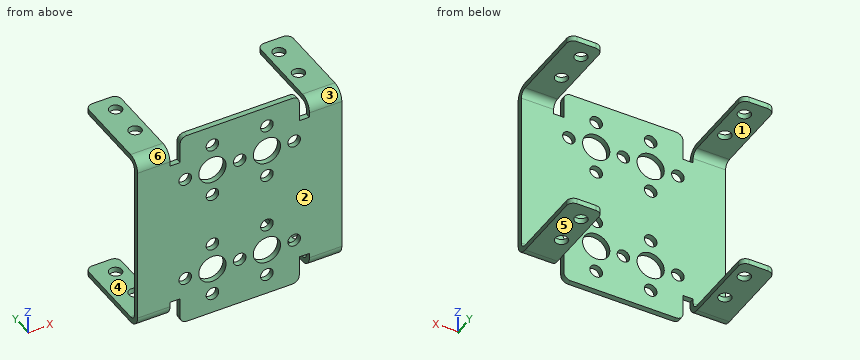
from build123d import *

# Parameters (mm, degrees)
BASE_FLANGE1_DEPTH             = 1.6
EDGE_FLANGE1_STRIP_W           = 10.4
EDGE_FLANGE1_STRIP_H           = 1.6
EDGE_FLANGE1_STRIP_CUT_DEPTH   = 9.5
EDGE_FLANGE1_STRIP_2_W         = 10.4
EDGE_FLANGE1_STRIP_2_H         = 1.6
EDGE_FLANGE1_STRIP_CUT_2_DEPTH = 9.5
EDGE_FLANGE1_DEPTH             = 9.5
EDGE_FLANGE1_BEND_DEPTH        = 9.5
CUT_EXTRUDE1_REACH             = 51.346
SKETCH15_R                     = 1.85
SKETCH15_R_2                   = 4
CUT_EXTRUDE2_REACH             = 50.448
SKETCH16_R                     = 1.85
FILLET1_R                      = 2


# Sheet-metal steps are written as plain solids
with BuildPart() as part:
    # Sketch1 → Base-Flange1 (new body)
    with BuildSketch(Plane(origin=(0, 0, 0), x_dir=(1, 0, 0), z_dir=(0, 1, 0))):
        Polygon((-30, 0), (30, 0), (30, -27), (20.5, -27), (20.5, -22), (17.5, -22), (17.5, -30), (-17.5, -30), (-17.5, -22), (-20.5, -22), (-20.5, -27), (-30, -27), align=None)
    extrude(amount=BASE_FLANGE1_DEPTH)

    # Edge-Flange1 strip (across the edge) → Edge-Flange1 strip cut (cut)
    with BuildSketch(Plane(origin=(20.5, 1.6, 27), x_dir=(0, 0, -1), z_dir=(1, 0, 0))):
        with Locations((-1.6, -0.8)):
            Rectangle(EDGE_FLANGE1_STRIP_W, EDGE_FLANGE1_STRIP_H)
    extrude(amount=EDGE_FLANGE1_STRIP_CUT_DEPTH, mode=Mode.SUBTRACT)

    # Edge-Flange1 strip 2 (across the edge) → Edge-Flange1 strip cut 2 (cut)
    with BuildSketch(Plane(origin=(-30, 1.6, 27), x_dir=(0, 0, -1), z_dir=(1, 0, 0))):
        with Locations((-1.6, -0.8)):
            Rectangle(EDGE_FLANGE1_STRIP_2_W, EDGE_FLANGE1_STRIP_2_H)
    extrude(amount=EDGE_FLANGE1_STRIP_CUT_2_DEPTH, mode=Mode.SUBTRACT)

    # Edge-Flange1 section (across the edge) → Edge-Flange1 (add)
    with BuildSketch(Plane(origin=(20.5, 1.6, 27), x_dir=(0, 0, -1), z_dir=(1, 0, 0))):
        with BuildLine():
            Line((0, 2), (0, 25.2))
            Line((0, 25.2), (1.6, 25.2))
            Line((1.6, 25.2), (1.6, 2))
            ThreePointArc((1.6, 2), (2.185786438, 0.585786438), (3.6, 0))
            Line((3.6, 0), (3.6, -1.6))
            ThreePointArc((3.6, -1.6), (1.054415588, -0.545584412), (0, 2))
        make_face()
    extrude(amount=EDGE_FLANGE1_DEPTH)

    # Edge-Flange1 section 2 (across the edge) → Edge-Flange1 bend (add)
    with BuildSketch(Plane(origin=(-30, 1.6, 27), x_dir=(0, 0, -1), z_dir=(1, 0, 0))):
        with BuildLine():
            Line((0, 2), (0, 25.2))
            Line((0, 25.2), (1.6, 25.2))
            Line((1.6, 25.2), (1.6, 2))
            ThreePointArc((1.6, 2), (2.185786438, 0.585786438), (3.6, 0))
            Line((3.6, 0), (3.6, -1.6))
            ThreePointArc((3.6, -1.6), (1.054415588, -0.545584412), (0, 2))
        make_face()
    extrude(amount=EDGE_FLANGE1_BEND_DEPTH)

    # Sketch15 → Cut-Extrude1 (cut, up to next)
    with BuildSketch(Plane(origin=(0, 1.6, 0), x_dir=(1, 0, 0), z_dir=(0, 1, 0)), mode=Mode.PRIVATE) as cut_extrude1_sk1:
        with Locations(Location((0, -16, 0), (0, 0, 270))):
            Circle(SKETCH15_R)
    cut_extrude1_tool1 = extrude(cut_extrude1_sk1.sketch, amount=-CUT_EXTRUDE1_REACH, mode=Mode.PRIVATE) & part.part
    # Sketch15 → Cut-Extrude1 (cut, up to next)
    with BuildSketch(Plane(origin=(0, 1.6, 0), x_dir=(1, 0, 0), z_dir=(0, 1, 0)), mode=Mode.PRIVATE) as cut_extrude1_sk2:
        with Locations(Location((8, -16, 0), (0, 0, 270))):
            Circle(SKETCH15_R_2)
    cut_extrude1_tool2 = extrude(cut_extrude1_sk2.sketch, amount=-CUT_EXTRUDE1_REACH, mode=Mode.PRIVATE) & part.part
    # Sketch15 → Cut-Extrude1 (cut, up to next)
    with BuildSketch(Plane(origin=(0, 1.6, 0), x_dir=(1, 0, 0), z_dir=(0, 1, 0)), mode=Mode.PRIVATE) as cut_extrude1_sk3:
        with Locations(Location((-8, -16, 0), (0, 0, 270))):
            Circle(SKETCH15_R_2)
    cut_extrude1_tool3 = extrude(cut_extrude1_sk3.sketch, amount=-CUT_EXTRUDE1_REACH, mode=Mode.PRIVATE) & part.part
    # Sketch15 → Cut-Extrude1 (cut, up to next)
    with BuildSketch(Plane(origin=(0, 1.6, 0), x_dir=(1, 0, 0), z_dir=(0, 1, 0)), mode=Mode.PRIVATE) as cut_extrude1_sk4:
        with Locations(Location((16, -16, 0), (0, 0, 270))):
            Circle(SKETCH15_R)
    cut_extrude1_tool4 = extrude(cut_extrude1_sk4.sketch, amount=-CUT_EXTRUDE1_REACH, mode=Mode.PRIVATE) & part.part
    # Sketch15 → Cut-Extrude1 (cut, up to next)
    with BuildSketch(Plane(origin=(0, 1.6, 0), x_dir=(1, 0, 0), z_dir=(0, 1, 0)), mode=Mode.PRIVATE) as cut_extrude1_sk5:
        with Locations(Location((-16, -16, 0), (0, 0, 270))):
            Circle(SKETCH15_R)
    cut_extrude1_tool5 = extrude(cut_extrude1_sk5.sketch, amount=-CUT_EXTRUDE1_REACH, mode=Mode.PRIVATE) & part.part
    # Sketch15 → Cut-Extrude1 (cut, up to next)
    with BuildSketch(Plane(origin=(0, 1.6, 0), x_dir=(1, 0, 0), z_dir=(0, 1, 0)), mode=Mode.PRIVATE) as cut_extrude1_sk6:
        with Locations(Location((-8, -8, 0), (0, 0, 270))):
            Circle(SKETCH15_R)
    cut_extrude1_tool6 = extrude(cut_extrude1_sk6.sketch, amount=-CUT_EXTRUDE1_REACH, mode=Mode.PRIVATE) & part.part
    # Sketch15 → Cut-Extrude1 (cut, up to next)
    with BuildSketch(Plane(origin=(0, 1.6, 0), x_dir=(1, 0, 0), z_dir=(0, 1, 0)), mode=Mode.PRIVATE) as cut_extrude1_sk7:
        with Locations(Location((-8, -24, 0), (0, 0, 270))):
            Circle(SKETCH15_R)
    cut_extrude1_tool7 = extrude(cut_extrude1_sk7.sketch, amount=-CUT_EXTRUDE1_REACH, mode=Mode.PRIVATE) & part.part
    # Sketch15 → Cut-Extrude1 (cut, up to next)
    with BuildSketch(Plane(origin=(0, 1.6, 0), x_dir=(1, 0, 0), z_dir=(0, 1, 0)), mode=Mode.PRIVATE) as cut_extrude1_sk8:
        with Locations(Location((8, -24, 0), (0, 0, 270))):
            Circle(SKETCH15_R)
    cut_extrude1_tool8 = extrude(cut_extrude1_sk8.sketch, amount=-CUT_EXTRUDE1_REACH, mode=Mode.PRIVATE) & part.part
    # Sketch15 → Cut-Extrude1 (cut, up to next)
    with BuildSketch(Plane(origin=(0, 1.6, 0), x_dir=(1, 0, 0), z_dir=(0, 1, 0)), mode=Mode.PRIVATE) as cut_extrude1_sk9:
        with Locations(Location((8, -8, 0), (0, 0, 270))):
            Circle(SKETCH15_R)
    cut_extrude1_tool9 = extrude(cut_extrude1_sk9.sketch, amount=-CUT_EXTRUDE1_REACH, mode=Mode.PRIVATE) & part.part
    add(cut_extrude1_tool1.solids().sort_by_distance((0, 1.6, 16))[0], mode=Mode.SUBTRACT)
    add(cut_extrude1_tool2.solids().sort_by_distance((8, 1.6, 16))[0], mode=Mode.SUBTRACT)
    add(cut_extrude1_tool3.solids().sort_by_distance((-8, 1.6, 16))[0], mode=Mode.SUBTRACT)
    add(cut_extrude1_tool4.solids().sort_by_distance((16, 1.6, 16))[0], mode=Mode.SUBTRACT)
    add(cut_extrude1_tool5.solids().sort_by_distance((-16, 1.6, 16))[0], mode=Mode.SUBTRACT)
    add(cut_extrude1_tool6.solids().sort_by_distance((-8, 1.6, 8))[0], mode=Mode.SUBTRACT)
    add(cut_extrude1_tool7.solids().sort_by_distance((-8, 1.6, 24))[0], mode=Mode.SUBTRACT)
    add(cut_extrude1_tool8.solids().sort_by_distance((8, 1.6, 24))[0], mode=Mode.SUBTRACT)
    add(cut_extrude1_tool9.solids().sort_by_distance((8, 1.6, 8))[0], mode=Mode.SUBTRACT)

    # Sketch16 → Cut-Extrude2 (cut, up to next)
    with BuildSketch(Plane.XY.offset(27), mode=Mode.PRIVATE) as cut_extrude2_sk1:
        with Locations((-24, 21.75)):
            Circle(SKETCH16_R)
    cut_extrude2_tool1 = extrude(cut_extrude2_sk1.sketch, amount=-CUT_EXTRUDE2_REACH, mode=Mode.PRIVATE) & part.part
    # Sketch16 → Cut-Extrude2 (cut, up to next)
    with BuildSketch(Plane.XY.offset(27), mode=Mode.PRIVATE) as cut_extrude2_sk2:
        with Locations((-24, 11.75)):
            Circle(SKETCH16_R)
    cut_extrude2_tool2 = extrude(cut_extrude2_sk2.sketch, amount=-CUT_EXTRUDE2_REACH, mode=Mode.PRIVATE) & part.part
    # Sketch16 → Cut-Extrude2 (cut, up to next)
    with BuildSketch(Plane.XY.offset(27), mode=Mode.PRIVATE) as cut_extrude2_sk3:
        with Locations((24, 21.75)):
            Circle(SKETCH16_R)
    cut_extrude2_tool3 = extrude(cut_extrude2_sk3.sketch, amount=-CUT_EXTRUDE2_REACH, mode=Mode.PRIVATE) & part.part
    # Sketch16 → Cut-Extrude2 (cut, up to next)
    with BuildSketch(Plane.XY.offset(27), mode=Mode.PRIVATE) as cut_extrude2_sk4:
        with Locations((24, 11.75)):
            Circle(SKETCH16_R)
    cut_extrude2_tool4 = extrude(cut_extrude2_sk4.sketch, amount=-CUT_EXTRUDE2_REACH, mode=Mode.PRIVATE) & part.part
    add(cut_extrude2_tool1.solids().sort_by_distance((-24, 21.75, 27))[0], mode=Mode.SUBTRACT)
    add(cut_extrude2_tool2.solids().sort_by_distance((-24, 11.75, 27))[0], mode=Mode.SUBTRACT)
    add(cut_extrude2_tool3.solids().sort_by_distance((24, 21.75, 27))[0], mode=Mode.SUBTRACT)
    add(cut_extrude2_tool4.solids().sort_by_distance((24, 11.75, 27))[0], mode=Mode.SUBTRACT)

    # Fillet1
    fillet1_edges = [part.edges().sort_by_distance(p)[0] for p in [
        (17.5, 0.8, 30),
        (-17.5, 0.8, 30),
        (20.5, 26.8, 26.2),
        (30, 26.8, 26.2),
        (-30, 26.8, 26.2),
        (-20.5, 26.8, 26.2),
    ]]
    fillet(fillet1_edges, radius=FILLET1_R)

    # Mirror1: part across plane


with BuildPart() as part_1:
    add(part.part)
    add(part.part.mirror(Plane(origin=(-30, 1.6, 0), x_dir=(1, 0, 0), z_dir=(0, 0, 1))))


solid = part_1.part
Model file for the job. Use its own axes, mm. Face numbers are marked on the shaded views. A direction names the side the tool comes from. Round coordinates to 2 decimals unless told otherwise and drop trailing zeros. Order: outer loops, then holes, each group sorted by start corner. A loop starts at its lowest first (then second) coordinate and runs counter-clockwise, first axis right, second up. Notation, with made-up numbers: M -1,-39 L 6,-39 A29 cw 6,-15 Z; hole C -2.75,-38 d2. An arc over 180 degrees is marked long. Write each question's results on one line, items separated by ' | '. Start each with the question number.
(1) Two-plate mould, pull along Z, no slides. Class the marked faces 1, 2 and 3: pulls with the +Z half, pulls with the -Z half, needs draft (parallel to the pull), parting line crosses it, or undercut.
(2) Saw through at B-B, the plane y = 5.5. Give the cut face in (x, z).
(3) Saw through at A-A, the plane y = 11.75. State how many separate pieces and enclosed holes the cut face has, then the cut area to 3 significant figures.
(4) Probe probe 1 along X at (y, z) = (0.75, -16); probe 2 along X at (y, z) = (1.2, 24); probe 3 along Z at (x, y) = (26, 10). List the from-to ranges inside material, lowest first. Write a range as from..to.
(5) Drop flat-ended pins along their axis: pin 1 (3 mm diameter, centred on x = 23.5, y = 20.5, fed in from +Z); pin 2 (9 mm diameter, centred on x = -8, z = 16, fed in from +Y); pin 3 (3 mm diameter, centred on x = 26.5, y = 20.5, fed in from -Z). Give the stop position or say it passes through.
(6) Saw through at D-D, the plane x = 13. Give the cut face in (y, z), then the cut area to 3 significant figures.
(7) Which spindle directions (+Z, -Z, +X, -X, +Y, -Y) get a long thin tool onto all of the face, cutting with end or side? Do the marked faces 4, 5 and 6. Say none if no direction does.
(8) Saw through at C-C, the plane z = -9. Give the cut face in (x, y).
Established:
1) face 1: undercut | face 2: needs draft | face 3: pulls with the +Z half
2) outline: M -30,-27 L -20.5,-27 L -20.5,-25.4 L -30,-25.4 Z; M -30,25.4 L -20.5,25.4 L -20.5,27 L -30,27 Z; M 20.5,-27 L 30,-27 L 30,-25.4 L 20.5,-25.4 Z; M 20.5,25.4 L 30,25.4 L 30,27 L 20.5,27 Z
3) separate pieces: 8 | enclosed holes: 0 | area: 37.1 mm^2
4) probe 1: x = -30..-17.85, -14.15..-12, -4..-1.85, 1.85..4, 12..14.15, 17.85..30 | probe 2: x = -30..-20.5, -17.5..-9.85, -6.15..6.15, 9.85..17.5, 20.5..30 | probe 3: z = -27..-25.4, 25.4..27
5) pin 1: stops at z = 27 | pin 2: stops at y = 1.6 | pin 3: stops at z = -27
6) outline: M 0,-30 L 1.6,-30 L 1.6,30 L 0,30 Z | area: 96.0 mm^2
7) face 4: +X, -X, +Y | face 5: -Z, +X, -X, +Y, -Y | face 6: +Z, -X, -Y
8) outline: M -30,0 L -9.56,0 L -9.56,1.6 L -30,1.6 Z; M -6.44,0 L 6.44,0 L 6.44,1.6 L -6.44,1.6 Z; M 9.56,0 L 30,0 L 30,1.6 L 9.56,1.6 Z
